Could you check a few things on this model? Use its own coordinates, in mm. Round coordinates to 2 decimals unless told otherwise and drop trailing zeros. Loops run counter-clockwise (first coordinate to the right, second up) from the corner with the lowest first, then second, coordinate; pieces in that order, holes last.
from build123d import *

# Parameters (mm, degrees)
F0_R     = 8.255
F1_DEPTH = 3.175
F2_DEPTH = 9.525
F3_D     = 12.7


with BuildPart() as f1:
    # F0 (on Front) → F1 (new body)
    with BuildSketch(Plane.XZ):
        with BuildLine():
            Line((92.999168, 15.848077), (-90.104167, 28.506954))
            ThreePointArc((-90.104167, 28.506954), (-120.65, 0), (-90.104167, -28.506954))
            Line((-90.104167, -28.506954), (92.999168, -15.848077))
            ThreePointArc((92.999168, -15.848077), (107.95, 0), (92.999168, 15.848077))
        make_face()
        with Locations((-92.075, 0)):
            Circle(F0_R, mode=Mode.SUBTRACT)
        with Locations((92.075, 0)):
            Circle(F0_R, mode=Mode.SUBTRACT)
    extrude(amount=F1_DEPTH)

    # F0 (on Front) → F2 (join)
    with BuildSketch(Plane.XZ):
        with Locations((-92.075, 0)):
            Circle(F0_R)
        with Locations((92.075, 0)):
            Circle(F0_R)
    extrude(amount=F2_DEPTH)

    # F3 (through all)
    with Locations(Plane(origin=(0, 0, 0), x_dir=(1, 0, 0), z_dir=(0, 1, 0))):
        with Locations((-92.075, 0), (92.075, 0)):
            Hole(F3_D / 2)


solid = f1.part
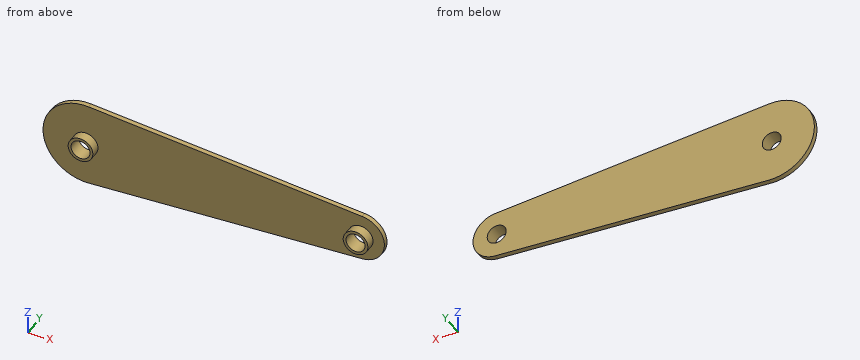
Item 1: If we section it at A-A, the plane z = 0: Please give me the cut outline in (x, y) (3 decimals).
Results list:
outline: (-120.65, -3.175) - (-100.33, -3.175) - (-100.33, -9.525) - (-98.425, -9.525) - (-98.425, 0) - (-120.65, 0) - close; (-85.725, -9.525) - (-83.82, -9.525) - (-83.82, -3.175) - (83.82, -3.175) - (83.82, -9.525) - (85.725, -9.525) - (85.725, 0) - (-85.725, 0) - close; (98.425, -9.525) - (100.33, -9.525) - (100.33, -3.175) - (107.95, -3.175) - (107.95, 0) - (98.425, 0) - close
Item 2: If we section it at C-C, the plane z = 18: Please give me the cut outline in (x, y) (3 decimals).
Results list:
outline: (-114.268, -3.175) - (61.873, -3.175) - (61.873, 0) - (-114.268, 0) - close
Item 3: Will these pins go through, and if not, where does the flat tip stop? pin 1 (12 mm diameter, centred on x = 0, z = -4.5, fed in from -Y) (3 decimals); pin 2 (4 mm diameter, centred on x = 5.5, y = -3, fed in from +Z).
Results list:
pin 1: stops at y = -3.175
pin 2: stops at z = 22.04
Item 4: If we section it at B-B, the plane x = -4: Please give me the cut outline in (y, z) (3 decimals), then the cut area to 3 significant figures.
Results list:
outline: (-3.175, -22.554) - (0, -22.554) - (0, 22.554) - (-3.175, 22.554) - close
area: 143 mm2
Item 5: If I drill on line 1 along Y through (x, z) = (64.5, 0.5) (3 decimals); line 2 along Z through (x, y) = (91, -6.75); line 3 along Z through (x, y) = (51, -0.75), over which ranges is the centre line in solid material (lowest first)?
Results list:
line 1: y = -3.175 to 0
line 2: z = -8.18 to -6.26, 6.26 to 8.18
line 3: z = -18.75 to 18.75
